Geometry check sheet. Reference: the model listing, model coordinates, mm. A direction names the side the tool comes from. Round coordinates to 2 decimals unless told otherwise and drop trailing zeros. Order: outer loops, then holes, each group sorted by start corner. A loop starts at its lowest first (then second) coordinate and runs counter-clockwise, first axis right, second up. Notation, with made-up numbers: (4.5, 76.25) - (43.5, 76.25) arc R10 ccw to (43.5, 87.25) - close; hole circle Ø7 at (4, 49). An arc over 180 degrees is marked (long way). Return JSON: item names as keys, results as strings. Group by question number.
Q1. Sectioned sample at D-D, the plane x = 14. Record the cut outline in (y, z).
Q2. Sectioned sample at C-C, the plane x = 0. Record the cut outline in (y, z).
Q3. Sectioned sample at A-A, the plane y = 0. Record the cut outline in (x, z) (1 decimal), then the cut area to 3 significant figures.
Q4. Material ranges on line 1 along X through (y, z) = (-4.75, 20) (1 decimal); line 2 along Y through (x, z) = (-6, 26.5); line 3 along Y through (x, z) = (0, 13), recorded low to high.
Q5. Tool access check on faces 4 (the flat face through (0, -7.938, 15)), 5 (the cylindrical face through (-25, 0, 15)), 6 (the cylindrical face through (25, 0, 15)), 7 (the flat face through (0, 7.938, 15)). Record the directions out of +Z, -Z, +X, -X, +Y, -Y that give a thin tool (end or side, any length) a straight path to the whole face; none if there is none.
Q6. Draft check along Y on faces 1 (the flat face through (6, 2, 35)), 2 (the cylindrical face through (13.066, 0.176, 17.255)), 3 (the conical face through (26.833, -0.215, 34.75)). Enter one of: pulls with the +Y half, pulls with the -Y half, needs draft (parallel to the pull), parting line crosses it, or undercut.
Q7. Sectioned sample at B-B, the plane z = 22. Record the cut outline in (x, y) (1 decimal), then the cut area to 3 significant figures.
Q8. Gauge pin test, flat ends, axial feed: pin 1 Ø1 at (x, y) = (19, -8.5) entering from -Z; pin 2 Ø4 at (x, y) = (-3, -2) entering from -Z; pin 3 Ø1.5 at (y, z) = (1, 5.5) entering from +X; pin 4 Ø1 at (x, z) = (18.5, 10) entering from +Y. Record the tip position at first contact, or that the pin passes through.
```python
from build123d import *

# Parameters (mm, degrees)
F0_R     = 5.9375
F0_R_2   = 5.9375000447
F0_R_3   = 4
F1_DEPTH = 30
F2_R     = 5.9375
F2_R_2   = 5.9375000447
F2_R_3   = 4
F3_DEPTH = 5
F4_SIZE2 = 4
F4_SIZE  = 2.3094010768


with BuildPart() as f1:
    # F0 (on Top) → F1 (new body)
    with BuildSketch(Plane.XY):
        with BuildLine():
            Line((-17.0625, -7.9375), (0, -7.9375))
            Line((0, -7.9375), (17.0625, -7.9375))
            ThreePointArc((17.0625, -7.9375), (25, 0), (17.0625, 7.9375))
            Line((17.0625, 7.9375), (0, 7.9375))
            Line((0, 7.9375), (-17.0625, 7.9375))
            ThreePointArc((-17.0625, 7.9375), (-25, 0), (-17.0625, -7.9375))
        make_face()
        with Locations((-17.0625, 0)):
            Circle(F0_R, mode=Mode.SUBTRACT)
        Circle(F0_R_2, mode=Mode.SUBTRACT)
        with Locations((17.0625, 0)):
            Circle(F0_R_3, mode=Mode.SUBTRACT)
    extrude(amount=F1_DEPTH)

    # F2 (on face) → F3 (join)
    with BuildSketch(Plane.XY.offset(30)):
        with BuildLine():
            ThreePointArc((17.0625, -11.9374991655), (28.9999991655, 0), (17.0625, 11.9374991655))
            Line((17.0625, 11.9374991655), (-17.0625, 11.9374991655))
            ThreePointArc((-17.0625, 11.9374991655), (-28.9999991655, 0), (-17.0625, -11.9374991655))
            Line((-17.0625, -11.9374991655), (17.0625, -11.9374991655))
        make_face()
        with BuildLine():
            ThreePointArc((-17.0625, -7.9375), (-25, 0), (-17.0625, 7.9375))
            Line((-17.0625, 7.9375), (17.0625, 7.9375))
            ThreePointArc((17.0625, 7.9375), (25, 0), (17.0625, -7.9375))
            Line((17.0625, -7.9375), (-17.0625, -7.9375))
        make_face(mode=Mode.SUBTRACT)
        with BuildLine():
            Line((17.0625, 7.9375), (-17.0625, 7.9375))
            ThreePointArc((-17.0625, 7.9375), (-25, 0), (-17.0625, -7.9375))
            Line((-17.0625, -7.9375), (17.0625, -7.9375))
            ThreePointArc((17.0625, -7.9375), (25, 0), (17.0625, 7.9375))
        make_face()
        with Locations((-17.0625, 0)):
            Circle(F2_R, mode=Mode.SUBTRACT)
        Circle(F2_R_2, mode=Mode.SUBTRACT)
        with Locations((17.0625, 0)):
            Circle(F2_R_3, mode=Mode.SUBTRACT)
    extrude(amount=F3_DEPTH)

    # F4
    f4_edges = [f1.edges().sort_by_distance(p)[0] for p in [
        (0, -11.937499, 35),
        (-28.999999, 0, 35),
        (0, 11.937499, 35),
        (28.999999, 0, 35),
    ]]
    f4_side = f1.faces().sort_by_distance((0, 11.310282, 35))[0]
    chamfer(f4_edges, length=F4_SIZE, length2=F4_SIZE2, reference=f4_side)


solid = f1.part
```
Reply:
{
 "1": {"outline": "(-11.94, 30) - (-7.94, 30) - (-7.94, 0) - (-2.57, 0) - (-2.57, 35) - (-9.63, 35) - (-11.94, 31) - close; (2.57, 0) - (7.94, 0) - (7.94, 30) - (11.94, 30) - (11.94, 31) - (9.63, 35) - (2.57, 35) - close"},
 "2": {"outline": "(-11.94, 30) - (-7.94, 30) - (-7.94, 0) - (-5.94, 0) - (-5.94, 35) - (-9.63, 35) - (-11.94, 31) - close; (5.94, 0) - (7.94, 0) - (7.94, 30) - (11.94, 30) - (11.94, 31) - (9.63, 35) - (5.94, 35) - close"},
 "3": {"outline": "(-29, 30) - (-25, 30) - (-25, 0) - (-23, 0) - (-23, 35) - (-26.7, 35) - (-29, 31) - close; (-11.1, 0) - (-5.9, 0) - (-5.9, 35) - (-11.1, 35) - close; (5.9, 0) - (13.1, 0) - (13.1, 35) - (5.9, 35) - close; (21.1, 0) - (25, 0) - (25, 30) - (29, 30) - (29, 31) - (26.7, 35) - (21.1, 35) - close", "area": "670 mm^2"},
 "4": {"line 1": "-23.4 to -20.6, -13.5 to -3.6, 3.6 to 23.4", "line 2": "-7.94 to 7.94", "line 3": "-7.94 to -5.94, 5.94 to 7.94"},
 "5": {"face 4": "-Z, +X, -X, -Y", "face 5": "-Z, -X", "face 6": "-Z, +X", "face 7": "-Z, +X, -X, +Y"},
 "6": {"face 1": "needs draft", "face 2": "undercut", "face 3": "parting line crosses it"},
 "7": {"outline": "(-17.1, -7.9) - (17.1, -7.9) arc R7.9 ccw to (17.1, 7.9) - (-17.1, 7.9) arc R7.9 ccw to start; hole circle Ø11.9 at (-17.1, 0); hole circle Ø11.9 at (0, 0); hole circle Ø8 at (17.1, 0)", "area": "468 mm^2"},
 "8": {"pin 1": "z = 30", "pin 2": "through", "pin 3": "x = 25", "pin 4": "y = 7.88"}
}
